from build123d import *

# Parameters (mm, degrees)
SKETCH1_W               = 50
SKETCH1_H               = 70
BOSS_EXTRUDE1_DEPTH     = 5
CUT_EXTRUDE2_START      = -2.5
CUT_EXTRUDE2_DEPTH      = 2.5
SKETCH5_W               = 5
SKETCH5_H               = 30
SKETCH5_W_2             = 15
SKETCH5_H_2             = 5
CUT_EXTRUDE3_DEPTH      = 1
CUT_EXTRUDE3_DEPTH_BACK = 6
SKETCH6_R               = 1.5875
CUT_EXTRUDE4_DEPTH      = 6


with BuildPart() as part:
    # Sketch1 → Boss-Extrude1 (new body)
    with BuildSketch(Plane(origin=(0, 0, 0), x_dir=(1, 0, 0), z_dir=(0, 1, 0))):
        with Locations((25, 35)):
            Rectangle(SKETCH1_W, SKETCH1_H)
    extrude(amount=BOSS_EXTRUDE1_DEPTH)

    # Sketch4 → Cut-Extrude2 (cut)
    with BuildSketch(Plane.XZ.offset(CUT_EXTRUDE2_START)):
        with BuildLine():
            Line((34.1625, -61), (15.8375, -61))
            ThreePointArc((15.8375, -61), (14.714967985, -60.535032015), (14.25, -59.4125))
            Line((14.25, -59.4125), (14.25, -43.0875))
            ThreePointArc((14.25, -43.0875), (14.714967985, -41.964967985), (15.8375, -41.5))
            Line((15.8375, -41.5), (34.1625, -41.5))
            ThreePointArc((34.1625, -41.5), (35.285032015, -41.964967985), (35.75, -43.0875))
            Line((35.75, -43.0875), (35.75, -59.4125))
            ThreePointArc((35.75, -59.4125), (35.285032015, -60.535032015), (34.1625, -61))
        make_face()
    extrude(amount=-CUT_EXTRUDE2_DEPTH, mode=Mode.SUBTRACT)

    # Sketch5 → Cut-Extrude3 (cut, two sides)
    with BuildSketch(Plane(origin=(0, 5, 0), x_dir=(1, 0, 0), z_dir=(0, 1, 0))) as cut_extrude3_sk:
        with Locations((2.5, 35)):
            Rectangle(SKETCH5_W, SKETCH5_H)
        with Locations((25, 67.5)):
            Rectangle(SKETCH5_W_2, SKETCH5_H_2)
        with Locations((47.5, 35)):
            Rectangle(SKETCH5_W, SKETCH5_H)
        with Locations((25, 2.5)):
            Rectangle(SKETCH5_W_2, SKETCH5_H_2)
    extrude(amount=CUT_EXTRUDE3_DEPTH, mode=Mode.SUBTRACT)
    extrude(cut_extrude3_sk.sketch, amount=-CUT_EXTRUDE3_DEPTH_BACK, mode=Mode.SUBTRACT)

    # Sketch6 → Cut-Extrude4 (cut, through all)
    with BuildSketch(Plane(origin=(0, 5, 0), x_dir=(1, 0, 0), z_dir=(0, 1, 0))):
        with Locations((5, 20)):
            Circle(SKETCH6_R)
        with Locations((5, 50)):
            Circle(SKETCH6_R)
        with Locations((17.5, 65)):
            Circle(SKETCH6_R)
        with Locations((32.5, 65)):
            Circle(SKETCH6_R)
        with Locations((45, 50)):
            Circle(SKETCH6_R)
        with Locations((45, 20)):
            Circle(SKETCH6_R)
        with Locations((32.5, 5)):
            Circle(SKETCH6_R)
        with Locations((17.5, 5)):
            Circle(SKETCH6_R)
        with Locations((17.5, 20)):
            Circle(SKETCH6_R)
        with Locations((32.5, 20)):
            Circle(SKETCH6_R)
    extrude(amount=-CUT_EXTRUDE4_DEPTH, mode=Mode.SUBTRACT)


solid = part.part
Source: CAD feature listing. Evaluate the final solid. Frame: model axes, mm. A direction names the side the tool comes from. Round coordinates to 2 decimals unless told otherwise and drop trailing zeros. Order: outer loops, then holes, each group sorted by start corner. A loop starts at its lowest first (then second) coordinate and runs counter-clockwise, first axis right, second up. Notation, with made-up numbers: (36, 69) - (84, 69) arc R18 ccw to (84, 97) - close; hole circle Ø11 at (55, 23.25). An arc over 180 degrees is marked (long way). Use a Markdown table: item, result. Add a question column.
1. Section query C-C (z = -47). Return the cut outline in (x, y), then the cut area to 3 significant figures.
2. Section query B-B (y = 1.5). Give the number of separate pieces and of enclosed holes in the cut face, then the cut area to 3 significant figures.
3. Section query D-D (z = -24). Return the cut outline in (x, y), then the cut area to 3 significant figures.
4. Mould query, pull axis Z, two halves, no side actions, for faces 4 (the flat face through (0, 2, -10)), 5 (the cylindrical face through (43.915, 2.535, -51.159)), 6 (the cylindrical face through (6.159, 2.535, -51.085)), 7 (the flat face through (25, 3, -65)). Classes: +Z half, -Z half, draft (parallel to the pull), parting line (faces both ways), or undercut.
5. Section query A-A (x = 26.5). Return the cut outline in (y, z).
6. Set-up query: faces 1 (the flat face through (17.5, 3, -2)), 2 (the flat face through (5, 3, -35)), 3 (the flat face through (32.5, 3, -68)). Return all of +Z, -Z, +X, -X, +Y, -Y with unobstructed straight access to the full face (end or side cutting, diameter ignored); none if empty.
7. First-contact query: pin 1 (4 mm diameter, centred on x = 32.5, z = -65, fed in from -Y); pin 2 (1.5 mm diameter, centred on y = 2, z = -39, fed in from -X); pin 3 (1.5 mm diameter, centred on y = 1, z = -29.5, fed in from +X); pin 4 (3 mm diameter, centred on x = 45, z = -20, fed in from +Y). Flat tips, straight axial feed; report the tip coordinate or a pass-through.
8. Line query: probe 1 along X at (y, z) = (1.15, -5.5); probe 2 along X at (y, z) = (2.6, -44); probe 3 along Y at (x, z) = (21, -60.5). Output: solid intervals per line, ascending.
Derived:
| question | item | result |
|---|---|---|
| 1 | outline | (5, 0) - (45, 0) - (45, 5) - (35.75, 5) - (35.75, 2.5) - (14.25, 2.5) - (14.25, 5) - (5, 5) - close |
| 1 | area | 146 mm2 |
| 2 | separate pieces | 1 |
| 2 | enclosed holes | 2 |
| 2 | area | 2,990 mm2 |
| 3 | outline | (5, 0) - (45, 0) - (45, 5) - (5, 5) - close |
| 3 | area | 200 mm2 |
| 4 | face 4 | draft |
| 4 | face 5 | undercut |
| 4 | face 6 | undercut |
| 4 | face 7 | -Z half |
| 5 | outline | (0, -65) - (5, -65) - (5, -61) - (2.5, -61) - (2.5, -41.5) - (5, -41.5) - (5, -5) - (0, -5) - close |
| 6 | face 1 | +Z, +Y, -Y |
| 6 | face 2 | -X, +Y, -Y |
| 6 | face 3 | -Z, +Y, -Y |
| 7 | pin 1 | y = 0 |
| 7 | pin 2 | x = 5 |
| 7 | pin 3 | x = 45 |
| 7 | pin 4 | through |
| 8 | probe 1 | 0 to 15.99, 19.01 to 30.99, 34.01 to 50 |
| 8 | probe 2 | 5 to 14.25, 35.75 to 45 |
| 8 | probe 3 | 0 to 2.5 |
